from build123d import *

# Parameters (mm, degrees)
SKETCH_1_R          = 1.5
SKETCH_1_R_2        = 2.1
EXTRUDE_1_DEPTH     = 55
FILLET_1_R          = 1
CUT_EXTRUDE_1_REACH = 99.788
SKETCH_2_W          = 29.048666984
SKETCH_2_H          = 34.015307271


with BuildPart() as part:
    # 草图1 → 凸台-拉伸1 (new, symmetric)
    with BuildSketch(Plane.XY):
        Polygon((-10, 10), (-10, 4.8), (-8.34, 3.14), (-8.34, 5.4), (-5.753553391, 5.4), (-3.8, 3.446446609), (-3.8, -3.446446609), (-5.753553391, -5.4), (-8.34, -5.4), (-8.34, -3.14), (-10, -4.8), (-10, -10), (-4.8, -10), (-3.14, -8.34), (-5.4, -8.34), (-5.4, -5.753553391), (-3.446446609, -3.8), (3.446446609, -3.8), (5.4, -5.753553391), (5.4, -8.34), (3.14, -8.34), (4.8, -10), (10, -10), (10, -4.8), (8.34, -3.14), (8.34, -5.4), (5.753553391, -5.4), (3.8, -3.446446609), (3.8, 3.446446609), (5.753553391, 5.4), (8.34, 5.4), (8.34, 3.14), (10, 4.8), (10, 10), (4.8, 10), (3.14, 8.34), (5.4, 8.34), (5.4, 5.753553391), (3.446446609, 3.8), (-3.446446609, 3.8), (-5.4, 5.753553391), (-5.4, 8.34), (-3.14, 8.34), (-4.8, 10), align=None)
        with Locations((-7.5, 7.5)):
            Circle(SKETCH_1_R, mode=Mode.SUBTRACT)
        Circle(SKETCH_1_R_2, mode=Mode.SUBTRACT)
        with Locations(Location((-7.5, -7.5, 0), (0, 0, 180))):
            Circle(SKETCH_1_R, mode=Mode.SUBTRACT)
        with Locations((7.5, -7.5)):
            Circle(SKETCH_1_R, mode=Mode.SUBTRACT)
        with Locations(Location((7.5, 7.5, 0), (0, 0, 180))):
            Circle(SKETCH_1_R, mode=Mode.SUBTRACT)
    extrude(amount=EXTRUDE_1_DEPTH, both=True)

    # 圆角1
    fillet_1_edges = [part.edges().sort_by_distance(p)[0] for p in [
        (10, 10, 0),
        (10, -10, 0),
        (-10, -10, 0),
        (-10, 10, 0),
    ]]
    fillet(fillet_1_edges, radius=FILLET_1_R)

    # 草图2 → 切除-拉伸1 (cut, up to next)
    with BuildSketch(Plane(origin=(-32.5, 0, -32.5), x_dir=(0, -1, 0), z_dir=(0.7071067811865464, 0, 0.7071067811865488)), mode=Mode.PRIVATE) as cut_extrude_1_sk1:
        with Locations((-4.05016126, 48.827458789)):
            Rectangle(SKETCH_2_W, SKETCH_2_H)
    cut_extrude_1_tool1 = extrude(cut_extrude_1_sk1.sketch, amount=CUT_EXTRUDE_1_REACH, mode=Mode.PRIVATE) & part.part
    cut_extrude_1 = cut_extrude_1_tool1.solids().sort_by_distance((2.026227, 4.050161, -67.026227))[0]
    add(cut_extrude_1, mode=Mode.SUBTRACT)

    # 镜向1: 切除-拉伸1 across plane
    add(cut_extrude_1.mirror(Plane(origin=(0, 0, 0), x_dir=(1, 0, 0), z_dir=(0, 0, -1))), mode=Mode.SUBTRACT)


solid = part.part
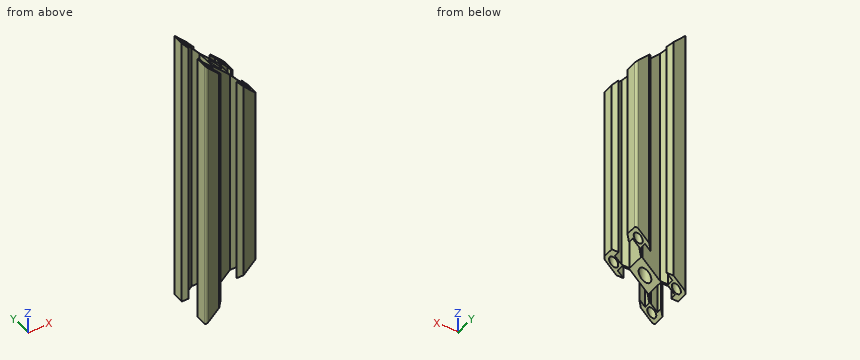
Source: CAD feature listing. Evaluate the final solid. Frame: model axes, mm. Give positions to 0.01 mm unless a question says otherwise; leave off trailing zeros. Write each loop counter-clockwise with the first axis right and the second up, starting at its lowest first coordinate (ties: lowest second). Pieces come first, ordered by that corner, then holes. Notation, with made-up numbers: M 71,42 L 102,42 A31 cw 102,72 Z; hole C 75.5,53 d4. An arc over 180 degrees is marked long. Return JSON: item names as keys, results as strings. Group by question number.
1) First-contact query: pin 1 Ø7.5 at (y, z) = (-0.5, -22) entering from -X; pin 2 Ø6.5 at (x, y) = (0, 0) entering from +Z; pin 3 Ø5.5 at (x, z) = (-1.5, 21) entering from +Y. Flat tips, straight axial feed; report the tip coordinate or a pass-through.
2) Ray query, L1, parallel to Y at x = -7.5, z = 30; L2, parallel to X at y = -7, z = 12. Return the intervals inside material, ascending.
3) Cut plane A-A, the plane x = 0. Output: boundary loops of the cut face in (y, z).
4) Cut plane B-B, the plane y = 0. Output: boundary loops of the cut face in (x, z).
5) Cut plane C-C, the plane z = 46. Give the number of separate pieces and of enclosed holes in the cut face, then the cut area to 3 significant figures.
Data:
{
 "1": {"pin 1": "stops at x = -9.45", "pin 2": "stops at z = 48.25", "pin 3": "stops at y = 9.45"},
 "2": {"L1": "y = -10 to -9, -6 to -5.4, 5.4 to 6, 9 to 10", "L2": "x = -10 to -8.91, -6.09 to -5.4, 5.4 to 6.09, 8.91 to 10"},
 "3": {"outline": "M -3.8,-45 L -2.1,-45 L -2.1,45 L -3.8,45 Z; M 2.1,-45 L 3.8,-45 L 3.8,45 L 2.1,45 Z"},
 "4": {"outline": "M -3.8,-48.8 L -2.1,-47.1 L -2.1,47.1 L -3.8,48.8 Z; M 2.1,-42.9 L 3.8,-41.2 L 3.8,41.2 L 2.1,42.9 Z"},
 "5": {"separate pieces": "1", "enclosed holes": "2", "area": "58.1 mm²"}
}
